Could you check a few things on this drawing? It's one solid part, dimensions in mm from its lowest x, y, z. Coordinates: 2 decimals unless noted, no trailing zeros. Write each loop counter-clockwise with the first axis right and the second up, starting at its lowest first coordinate (ties: lowest second). Pieces come first, ordered by that corner, then holes. Notation, with made-up numbers: M 78,53.5 L 131,53.5 A14 cw 131,63.5 Z; hole C -1,2.5 d11. An arc over 180 degrees is marked long. Use a Markdown table: item, result.
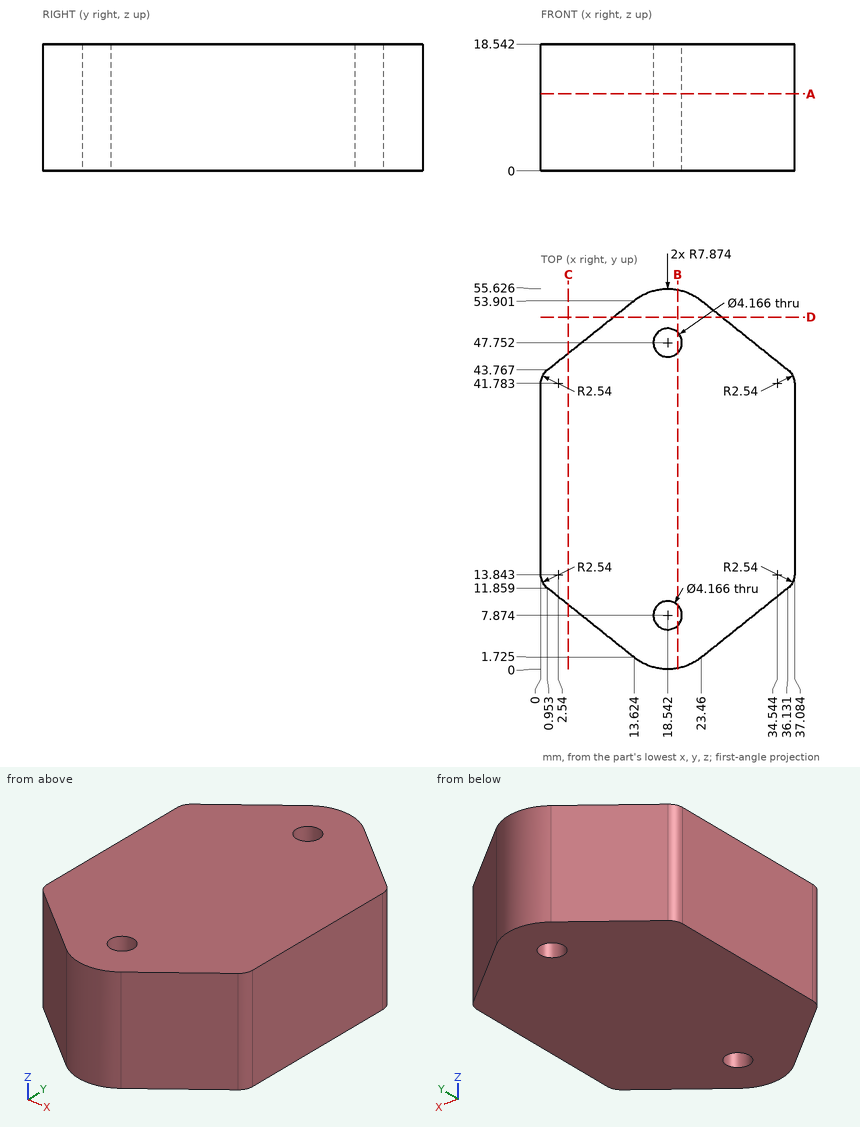
1. Suppose I cut it at D-D on y = 51.5. Write out the boundary of the cut face in (x, z), and give its area (3 significant figures).
Answers follow:
| item | result |
|---|---|
| outline | M 10.62,0 L 26.46,0 L 26.46,18.54 L 10.62,18.54 Z |
| area | 294 mm2 |
2. Suppose I cut it at A-A on z = 11.25. Write out the boundary of the cut face in (x, y) (1 decimal).
Answers follow:
| item | result |
|---|---|
| outline | M 0,13.8 A2.5 ccw 1,11.9 L 13.6,1.7 A7.9 ccw 23.5,1.7 L 36.1,11.9 A2.5 ccw 37.1,13.8 L 37.1,41.8 A2.5 ccw 36.1,43.8 L 23.5,53.9 A7.9 ccw 13.6,53.9 L 1,43.8 A2.5 ccw 0,41.8 Z; hole C 18.5,7.9 d4.2; hole C 18.5,47.8 d4.2 |
3. Suppose I cut it at B-B on x = 20. Write out the boundary of the cut face in (y, z) (1 decimal), and give its area (3 significant figures).
Answers follow:
| item | result |
|---|---|
| outline | M 0.1,0 L 6.4,0 L 6.4,18.5 L 0.1,18.5 Z; M 9.4,0 L 46.3,0 L 46.3,18.5 L 9.4,18.5 Z; M 49.2,0 L 55.5,0 L 55.5,18.5 L 49.2,18.5 Z |
| area | 916 mm2 |
4. Suppose I cut it at C-C on x = 4. Write out the boundary of the cut face in (y, z).
Answers follow:
| item | result |
|---|---|
| outline | M 9.42,0 L 46.2,0 L 46.2,18.54 L 9.42,18.54 Z |
5. Will these pins go through, and if not, where does the flat tip stop? pin 1 Ø2 at (x, z) = (11.5, 3) entering from -Y (1 decimal); pin 2 Ø1.5 at (x, z) = (4, 6.5) entering from -Y; pin 3 Ø2 at (y, z) = (7.5, 14) entering from -X (1 decimal).
Answers follow:
| item | result |
|---|---|
| pin 1 | stops at y = 2.6 |
| pin 2 | stops at y = 8.82 |
| pin 3 | stops at x = 5.2 |
6. I need wall thicknesses on probe 1 along X at (y, z) = (8.5, 4.5) (1 decimal); probe 2 along Y at (x, z) = (12.5, 13.75) (1 decimal); probe 3 along Y at (x, z) = (21, 16) (1 decimal). Which ranges of each line are inside material? Lowest first, please.
Answers follow:
| item | result |
|---|---|
| probe 1 | x = 5.2 to 16.6, 20.5 to 31.9 |
| probe 2 | y = 2.6 to 53 |
| probe 3 | y = 0.4 to 55.2 |
